Geometry check sheet. Reference: the model listing, model coordinates, mm. Face numbers are marked on the shaded views. A direction names the side the tool comes from. Give positions to 0.01 mm unless a question says otherwise; leave off trailing zeros. Loops run counter-clockwise (first coordinate to the right, second up) from the corner with the lowest first, then second, coordinate; pieces in that order, holes last. Notation, with made-up numbers: (39.5, 44) -> (65.5, 44) arc R15 cw to (65.5, 55) -> close; hole circle Ø7 at (15.25, -27). An arc over 180 degrees is marked (long way). One line per item, written item: value. Start each with the question number.
(1) Gauge pin test, flat ends, axial feed: pin 1 Ø5 at (x, z) = (-46, 28) entering from -Y; pin 2 Ø9 at (x, z) = (-34.5, 15.5) entering from -Y; pin 3 Ø2.5 at (y, z) = (28, 16) entering from -X; pin 4 Ø2.5 at (x, y) = (-20.5, 5.5) entering from -Z. Record the tip position at first contact, or that the pin passes through.
(2) Scan lines: line 1 along Y through (x, z) = (-19, 14.5); line 2 along Y through (x, z) = (-20.5, 12.75); line 3 along Z through (x, y) = (-11.5, 38). Record each from-to range of solid material in increasing order. Write a range as from..to.
(3) Sectioned sample at A-A, the plane x = -26. Record the cut outline in (y, z).
(4) Sectioned sample at C-C, the plane y = 36.5. Record the cut outline in (x, z).
(5) Tool access check on the marked faces 1, 2, 3, 4 and 5. Record the directions out of +Z, -Z, +X, -X, +Y, -Y that give a thin tool (end or side, any length) a straight path to the whole face; none if there is none.
(6) Sectioned sample at B-B, the plane z = 13. Record the cut outline in (x, y), then the cut area to 3 significant figures.
(7) Sectioned sample at D-D, the plane y = 46. Record the cut outline in (x, z), then the cut area to 3 significant figures.
(8) Draft check along Y on the marked faces 6, 7, 8 and 9. Enter one of: pulls with the +Y half, pulls with the -Y half, needs draft (parallel to the pull), parting line crosses it, or undercut.
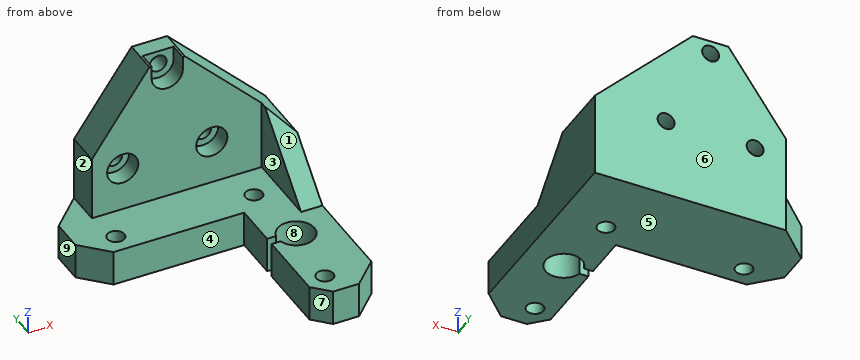
from build123d import *

# Parameters (mm, degrees)
SKETCH_R        = 1.9
SKETCH_R_2      = 4.1
PAD_DEPTH       = 8
PAD001_DEPTH    = 33
SKETCH002_R     = 1.9
POCKET_DEPTH    = 7.801
POCKET001_DEPTH = 5
POCKET002_DEPTH = 52.001
SKETCH006_R     = 3.5
POCKET003_DEPTH = 4
SKETCH007_W     = 2.023821
SKETCH007_H     = 2
POCKET004_DEPTH = 8.001


with BuildPart() as pocket004:
    # Sketch → Pad (new body)
    with BuildSketch(Plane.XY.offset(10)):
        Polygon((0, 52), (0, 5.656854), (5.656854, 0), (11.464466, 0), (15, 3.535534), (15, 32), (44.343146, 32), (50, 37.656854), (50, 44.928932), (42.928932, 52), align=None)
        with Locations((41.5, 36.5)):
            Circle(SKETCH_R, mode=Mode.SUBTRACT)
        with Locations((10.5, 36.5)):
            Circle(SKETCH_R, mode=Mode.SUBTRACT)
        with Locations((10.5, 5.5)):
            Circle(SKETCH_R, mode=Mode.SUBTRACT)
        with Locations((9, 21)):
            Circle(SKETCH_R_2, mode=Mode.SUBTRACT)
    extrude(amount=PAD_DEPTH)

    # Sketch001 → Pad001 (new body)
    with BuildSketch(Plane.XY.offset(18)):
        Polygon((42.928932, 52), (0, 52), (0, 27), (4.8, 27), (4.8, 44.2), (42.928932, 44.2), align=None)
    extrude(amount=PAD001_DEPTH)

    # Sketch002 → Pocket (cut, through all)
    with BuildSketch(Plane(origin=(0, 44.2, 10), x_dir=(1, 0, 0), z_dir=(0, -1, 0))):
        with Locations((26, 38)):
            Circle(SKETCH002_R)
        with Locations((16, 18)):
            Circle(SKETCH002_R)
        with Locations((36, 18)):
            Circle(SKETCH002_R)
    extrude(amount=-POCKET_DEPTH, mode=Mode.SUBTRACT)

    # Sketch003 → Pocket001 (cut)
    with BuildSketch(Plane(origin=(4.8, 0, 10), x_dir=(0, 1, 0), z_dir=(1, 0, 0))):
        Polygon((27, 8), (44.2, 25.2), (44.2, 41), (27, 41), align=None)
    extrude(amount=-POCKET001_DEPTH, mode=Mode.SUBTRACT)

    # Sketch005 → Pocket002 (cut, through all)
    with BuildSketch(Plane(origin=(0, 52, 10), x_dir=(-1, 0, 0), z_dir=(0, 1, 0))):
        Polygon((-42.928932, 22.535571), (-30, 41), (-42.928932, 41), align=None)
        Polygon((-22, 41), (0, 19), (0, 41), align=None)
    extrude(amount=-POCKET002_DEPTH, mode=Mode.SUBTRACT)

    # Sketch006 → Pocket003 (cut)
    with BuildSketch(Plane(origin=(0, 44.2, 10), x_dir=(1, 0, 0), z_dir=(0, -1, 0))):
        with Locations((16, 18)):
            Circle(SKETCH006_R)
        with Locations((36, 18)):
            Circle(SKETCH006_R)
        with BuildLine():
            ThreePointArc((22.5, 38), (26, 34.5), (29.5, 38))
            Line((29.5, 41), (29.5, 38))
            Line((22.5, 41), (29.5, 41))
            Line((22.5, 38), (22.5, 41))
        make_face()
    extrude(amount=-POCKET003_DEPTH, mode=Mode.SUBTRACT)

    # Sketch007 → Pocket004 (cut, through all)
    with BuildSketch(Plane.XY.offset(18)):
        with Locations((13.98809, 21)):
            Rectangle(SKETCH007_W, SKETCH007_H)
    extrude(amount=-POCKET004_DEPTH, mode=Mode.SUBTRACT)


with BuildPart() as part_mirroring:
    # Part__Mirroring: instance of Pocket004
    add(pocket004.part.mirror(Plane(origin=(0, 26, 30.500002), x_dir=(0, -1, 0), z_dir=(1, 0, 0))))


with BuildPart() as part_mirroring_1:
    # Part__Mirroring placement: moved
    add(part_mirroring.part.moved(Location((-10, 0, 0))))


solid = part_mirroring_1.part
Calculated:
1. pin 1: stops at y = 48.2
1. pin 2: stops at y = 32
1. pin 3: stops at x = -25
1. pin 4: passes through
2. line 1: y = 0..4.33, 6.67..16.9, 25.1..35.33, 37.67..52
2. line 2: y = 0..3.6, 7.4..17.18, 24.82..34.6, 38.4..52
2. line 3: z = 10..29
3. outline: (32, 10) -> (52, 10) -> (52, 26.1) -> (48.2, 26.1) -> (48.2, 24.5) -> (44.2, 24.5) -> (44.2, 18) -> (32, 18) -> close; (44.2, 31.5) -> (48.2, 31.5) -> (48.2, 29.9) -> (52, 29.9) -> (52, 45) -> (44.2, 45) -> close
4. outline: (-58.84, 10) -> (-53.4, 10) -> (-53.4, 18) -> (-58.84, 18) -> close; (-49.6, 10) -> (-22.4, 10) -> (-22.4, 18) -> (-49.6, 18) -> close; (-18.6, 10) -> (-10, 10) -> (-10, 27.5) -> (-14.8, 27.5) -> (-14.8, 18) -> (-18.6, 18) -> close
5. face 1: +Z, +X, -X, -Y
5. face 2: +Z, -X, +Y, -Y
5. face 3: +Z, -X, -Y
5. face 4: +Z, -Z, -X, -Y
5. face 5: -Z, +X, -X, +Y, -Y
6. outline: (-60, 37.66) -> (-54.34, 32) -> (-25, 32) -> (-25, 22) -> (-22.98, 22) arc R4.1 cw (long way) to (-22.98, 20) -> (-25, 20) -> (-25, 3.54) -> (-21.46, 0) -> (-15.66, 0) -> (-10, 5.66) -> (-10, 52) -> (-52.93, 52) -> (-60, 44.93) -> close; hole circle Ø3.8 at (-51.5, 36.5); hole circle Ø3.8 at (-20.5, 5.5); hole circle Ø3.8 at (-20.5, 36.5)
6. area: 1,330 mm2
7. outline: (-58.93, 10) -> (-10, 10) -> (-10, 29) -> (-32, 51) -> (-32.5, 51) -> (-32.5, 48) arc R3.5 cw to (-39.5, 48) -> (-39.5, 51) -> (-40, 51) -> (-52.93, 32.54) -> (-52.93, 18) -> (-58.93, 18) -> close; hole circle Ø7 at (-46, 28); hole circle Ø7 at (-26, 28)
7. area: 1,330 mm2
8. face 6: pulls with the +Y half
8. face 7: pulls with the -Y half
8. face 8: undercut
8. face 9: needs draft
